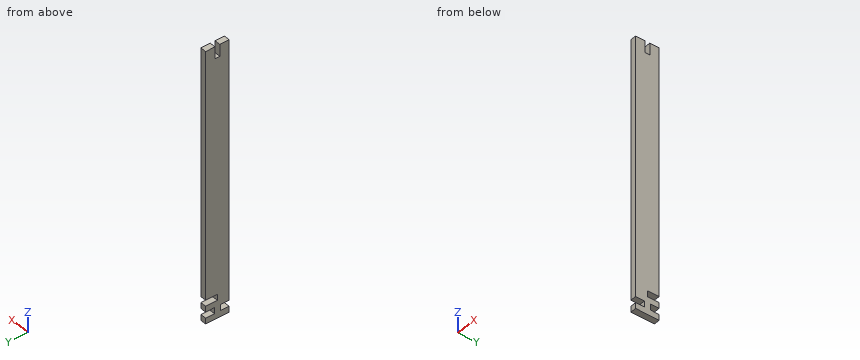
```python
from build123d import *

# Parameters (mm, degrees)
PAD_DEPTH = 2.5


with BuildPart() as part:
    # Sketch → Pad (new body, symmetric)
    with BuildSketch(Plane.YZ):
        Polygon((10, 0), (10, 4.95), (2.5, 4.95), (2.5, 10.05), (10, 10.05), (10, 14.95), (0, 14.95), (0, 20.05), (10, 20.05), (10, 230), (2.05, 230), (2.05, 220), (-2.05, 220), (-2.05, 230), (-10, 230), (-10, 10.05), (-2.5, 10.05), (-2.5, 4.95), (-10, 4.95), (-10, 0), align=None)
    extrude(amount=PAD_DEPTH, both=True)


solid = part.part
```
Input: part model. Units: mm. Frame: model coordinates. Round coordinates to 2 decimals unless told otherwise and drop trailing zeros. Order: outer loops, then holes, each group sorted by start corner. A loop starts at its lowest first (then second) coordinate and runs counter-clockwise, first axis right, second up. Notation, with made-up numbers: (-25, -21.75) - (17, -21.75) arc R10 ccw to (17, -3.75) - close; hole circle Ø11 at (51, 3.25). An arc over 180 degrees is marked (long way). Answer in a Markdown table with one row per item.
Item 1: Section query A-A (y = -5.5). Return the cut outline in (x, z), then the cut area to 3 significant figures.
Model answer:
| item | result |
|---|---|
| outline | (-2.5, 0) - (2.5, 0) - (2.5, 4.95) - (-2.5, 4.95) - close; (-2.5, 10.05) - (2.5, 10.05) - (2.5, 230) - (-2.5, 230) - close |
| area | 1,120 mm² |
Item 2: Pin query (flat end, axial travel): pin 1 (2.5 mm diameter, centred on x = -0.5, z = 18.5, fed in from +Y); pin 2 (2.5 mm diameter, centred on x = 0, z = 8, fed in from -Y); pin 3 (2 mm diameter, centred on x = 0, y = 0.5, fed in from +Z). Return the tip coordinate at first contact, or that it passes through.
Model answer:
| item | result |
|---|---|
| pin 1 | stops at y = 0 |
| pin 2 | stops at y = -2.5 |
| pin 3 | stops at z = 220 |
Item 3: Line query: line 1 (Z direction, x = 1.25, y = 3.25); line 2 (Z direction, x = 1.1, y = -8.25); line 3 (Z direction, x = 0.2, y = 1.5). Output: solid intervals per line, ascending.
Model answer:
| item | result |
|---|---|
| line 1 | z = 0 to 4.95, 10.05 to 14.95, 20.05 to 230 |
| line 2 | z = 0 to 4.95, 10.05 to 230 |
| line 3 | z = 0 to 14.95, 20.05 to 220 |
Item 4: Section query B-B (x = 0.7). Return the cut outline in (y, z).
Model answer:
| item | result |
|---|---|
| outline | (-10, 0) - (10, 0) - (10, 4.95) - (2.5, 4.95) - (2.5, 10.05) - (10, 10.05) - (10, 14.95) - (0, 14.95) - (0, 20.05) - (10, 20.05) - (10, 230) - (2.05, 230) - (2.05, 220) - (-2.05, 220) - (-2.05, 230) - (-10, 230) - (-10, 10.05) - (-2.5, 10.05) - (-2.5, 4.95) - (-10, 4.95) - close |
